Autodesk Inventor part; units mm, degrees
ref_plane "YZ Plane" through (0, 0, 0) normal (1, 0, 0) x (0, 1, 0)
ref_plane "XZ Plane" through (0, 0, 0) normal (0, 1, 0) x (-1, 0, 0)
ref_plane "XY Plane" through (0, 0, 0) normal (0, 0, 1) x (1, 0, 0)
sketch "Sketch1" plane through (0, 0, 0) normal (0, 0, 1) x (1, 0, 0)
  line L0 (0, 0) -> (25.4, 0)
  line L1 (25.4, 0) -> (25.4, 25.4)
  line L2 (25.4, 25.4) -> (0, 25.4)
  line L3 (0, 25.4) -> (0, 0)
  dimension "d0" = 25.4
  dimension "d1" = 25.4
extrude "Extrusion1" add sketch "Sketch1" along normal blind 457.2
shell "Shell1" thickness 2.54 removed faces 2 at (8.4667, 16.9333, 0) at (8.4667, 16.9333, 457.2)
sketch "Sketch2" plane through (0, 25.4, 0) normal (0, 1, 0) x (1, 0, 0)
  line L0 (25.4, 0) -> (0, 0)
  line L1 (0, 0) -> (0, -457.2)
  point P0 (12.7, -12.7)
  point P1 (12.7, -38.1)
  point P2 (12.7, -63.5)
  point P3 (12.7, -88.9)
  point P4 (12.7, -114.3)
  point P5 (12.7, -139.7)
  point P6 (12.7, -165.1)
  point P7 (12.7, -190.5)
  point P8 (12.7, -215.9)
  point P9 (12.7, -241.3)
  point P10 (12.7, -266.7)
  point P11 (12.7, -292.1)
  point P12 (12.7, -317.5)
  point P13 (12.7, -342.9)
  point P14 (12.7, -368.3)
  point P15 (12.7, -393.7)
  point P16 (12.7, -419.1)
  point P17 (12.7, -444.5)
  point P18 (12.7, -469.9)
  point P19 (12.7, -495.3)
  point P20 (12.7, -520.7)
  point P21 (12.7, -546.1)
  point P22 (12.7, -571.5)
  point P23 (12.7, -596.9)
  point P24 (12.7, -622.3)
  point P25 (12.7, -647.7)
  point P26 (12.7, -673.1)
  point P27 (12.7, -698.5)
  point P28 (12.7, -723.9)
  point P29 (12.7, -749.3)
  point P30 (12.7, -774.7)
  point P31 (12.7, -800.1)
  point P32 (12.7, -825.5)
  point P33 (12.7, -850.9)
  point P34 (12.7, -876.3)
  point P35 (12.7, -901.7)
  point P36 (12.7, -927.1)
  dimension "d5" = 12.7
  dimension "d6" = 12.7
  dimension "d9" = 25.4
hole "Hole1" at (12.7, 25.4, 12.7) at (12.7, 25.4, 38.1) at (12.7, 25.4, 63.5) at (12.7, 25.4, 88.9) at (12.7, 25.4, 114.3) at (12.7, 25.4, 139.7) at (12.7, 25.4, 165.1) at (12.7, 25.4, 190.5) at (12.7, 25.4, 215.9) at (12.7, 25.4, 241.3) at (12.7, 25.4, 266.7) at (12.7, 25.4, 292.1) at (12.7, 25.4, 317.5) at (12.7, 25.4, 342.9) at (12.7, 25.4, 368.3) at (12.7, 25.4, 393.7) at (12.7, 25.4, 419.1) at (12.7, 25.4, 444.5) at (12.7, 25.4, 469.9) at (12.7, 25.4, 495.3) at (12.7, 25.4, 520.7) at (12.7, 25.4, 546.1) at (12.7, 25.4, 571.5) at (12.7, 25.4, 596.9) at (12.7, 25.4, 622.3) at (12.7, 25.4, 647.7) at (12.7, 25.4, 673.1) at (12.7, 25.4, 698.5) at (12.7, 25.4, 723.9) at (12.7, 25.4, 749.3) at (12.7, 25.4, 774.7) at (12.7, 25.4, 800.1) at (12.7, 25.4, 825.5) at (12.7, 25.4, 850.9) at (12.7, 25.4, 876.3) at (12.7, 25.4, 901.7) direction (0, -1, 0) diameter 2.54 depth 50.8 tip angle 118
properties part number "cross bar" material "Aluminum 6061"
Build history of the part. All positions in model axes, mm. A direction names the side the tool comes from. Coordinates: 2 decimals unless noted, no trailing zeros. Order: outer loops, then holes, each group sorted by start corner. A loop starts at its lowest first (then second) coordinate and runs counter-clockwise, first axis right, second up. Notation, with made-up numbers: (58, 21) -> (92, 21) arc R25 cw to (92, 43) -> close; hole circle Ø7 at (50.25, 7). An arc over 180 degrees is marked (long way). Answer in a Markdown table with one row per item. Add a question column.
Q1. Mould opens along Y. For faces 3 (the face through (13, 22.86, 225)), 4 (the face through (13, 25.4, 225)), 5 (the face through (22.86, 13, 225)), 6 (the face through (13, 0, 225)) say: +Y half, -Y half, draft (parallel to the pull), parting line (faces both ways), or undercut.
Q2. Drop flat-ended pins along their axis: pin 1 (10 mm diameter, centred on y = 15.5, z = 214.5, fed in from -X); pin 2 (1.5 mm diameter, centred on x = 12.7, z = 292.1, fed in from +Y). Give the stop position or say it passes through.
Q3. Wall check: line 1 along Y through (x, z) = (20.5, 138.5); line 2 along X through (y, z) = (24.75, 368.3). Give the ranges that are in metal, low to high. Write a range as [from, to].
Q4. Band-saw the part on C-C, the plane z = 200.5. List the corners of the cut face in (x, y).
Q5. Band-saw the part on A-A, the plane x = 6.25. List the corners of the cut face in (y, z), then the cut area to 3 significant figures.
Q6. Which spindle directions (+Z, -Z, +X, -X, +Y, -Y) get a long thin tool onto all of the face, cutting with end or side? Do faces 1 (the face through (25.4, 13, 225)), 2 (the face through (13, 2.54, 225)). Say none if no direction does.
Answers follow:
| question | item | result |
|---|---|---|
| 1 | face 3 | undercut |
| 1 | face 4 | +Y half |
| 1 | face 5 | undercut |
| 1 | face 6 | -Y half |
| 2 | pin 1 | x = 0 |
| 2 | pin 2 | through |
| 3 | line 1 | [0, 2.54], [22.86, 25.4] |
| 3 | line 2 | [0, 11.43], [13.97, 25.4] |
| 4 | outline | (0, 0) -> (25.4, 0) -> (25.4, 25.4) -> (0, 25.4) -> close; hole (2.54, 2.54) -> (22.86, 2.54) -> (22.86, 22.86) -> (2.54, 22.86) -> close |
| 5 | outline | (0, 0) -> (2.54, 0) -> (2.54, 457.2) -> (0, 457.2) -> close; (22.86, 0) -> (25.4, 0) -> (25.4, 457.2) -> (22.86, 457.2) -> close |
| 5 | area | 2,320 mm^2 |
| 6 | face 1 | +Z, -Z, +X, +Y, -Y |
| 6 | face 2 | +Z, -Z |
